Input: part model. Units: mm. Frame: model coordinates. Face numbers are marked on the shaded views. Coordinates: 2 decimals unless noted, no trailing zeros. Loops run counter-clockwise (first coordinate to the right, second up) from the corner with the lowest first, then second, coordinate; pieces in that order, holes last. Notation, with made-up numbers: (25, -26.5) - (34, -26.5) arc R10 ccw to (34, -12.5) - close; hole circle Ø2 at (88, -26). An arc over 180 degrees is marked (long way). Use a Markdown table: item, result. Add a question column.
1. Contact query for flat-ended pins moving along their axis: P1, Ø12.5, axis at x = 163, z = 273, coming from the -Y side; P2, Ø12.5, axis at y = -340.5, z = 255, coming from the -X side; P3, Ø20.5, axis at y = -67.5, z = 149, coming from the +X side; P4, Ø15, axis at x = 212.5, y = -168, coming from the +Z side. Output: stop coordinate, or through.
2. Section query B-B on x = 169.5. Return the cut outline in (y, z).
3. Section query A-A on z = 201.5. Return the cut outline in (x, y), then the cut area to 3 significant figures.
4. Ray query, L1, parallel to Z at x = 201, y = -199; L2, parallel to Y at x = 237.5, z = 107. Return the intervals inside material, ascending. Write a range as [from, to].
5. Draft query along X for the marked faces 1, 2 and 3. Return one class per face: released by +X, released by -X, zero draft, split by the parting line, or undercut.
Autodesk Inventor part; units mm, degrees
ref_plane "YZ Plane" through (0, 0, 0) normal (1, 0, 0) x (0, 1, 0)
ref_plane "XZ Plane" through (0, 0, 0) normal (0, 1, 0) x (-1, 0, 0)
ref_plane "XY Plane" through (0, 0, 0) normal (0, 0, 1) x (1, 0, 0)
sketch "Sketch1" plane through (0, 0, 0) normal (0, 0, 1) x (1, 0, 0)
  line L0 (0, 0) -> (812.8, 0) construction
  line L1 (812.8, 0) -> (812.8, -406.4) construction
  line L2 (812.8, -406.4) -> (0, -406.4) construction
  line L3 (0, -406.4) -> (0, 0) construction
  line L4 (0, 0) -> (406.4, 0)
  line L5 (406.4, 0) -> (406.4, -25.4)
  line L6 (406.4, -25.4) -> (0, -25.4)
  line L7 (0, -25.4) -> (0, 0)
  line L8 (406.4, -25.4) -> (381, -25.4)
  line L9 (381, -25.4) -> (381, -406.4)
  line L10 (381, -406.4) -> (406.4, -406.4)
  line L11 (406.4, -406.4) -> (406.4, -25.4)
  line L12 (381, -406.4) -> (0, -406.4)
  line L13 (0, -406.4) -> (0, -381)
  line L14 (0, -381) -> (381, -381)
  line L15 (381, -381) -> (381, -406.4)
  line L16 (0, -381) -> (25.4, -381)
  line L17 (25.4, -381) -> (25.4, -25.4)
  line L18 (25.4, -25.4) -> (0, -25.4)
  line L19 (0, -25.4) -> (0, -381)
  dimension "d1" = 812.8
  dimension "d5" = 406.4
  dimension "d6" = 25.4
  dimension "d7" = 25.4
  dimension "d8" = 381
  dimension "d9" = 381
  dimension "d10" = 25.4
  dimension "d11" = 25.4
extrude "Extrusion1" add sketch "Sketch1" against normal blind 25.4 contours L6 L9 L14 L17
sketch "Sketch3" plane through (0, 0, 0) normal (0, 0, 1) x (1, 0, 0)
  line L0 (-406.4, 0) -> (406.4, 0) construction
  line L1 (406.4, 0) -> (406.4, -406.4) construction
  line L2 (406.4, -406.4) -> (-406.4, -406.4) construction
  line L3 (-406.4, -406.4) -> (-406.4, 0) construction
  line L4 (406.4, -406.4) -> (406.4, 0)
  line L5 (381, -381) -> (25.4, -381)
  line L6 (25.4, -381) -> (177.8, -381)
  line L7 (177.8, -381) -> (203.2, -381)
  line L8 (177.8, -381) -> (177.8, -355.6)
  line L9 (177.8, -355.6) -> (228.6, -355.6)
  line L10 (228.6, -355.6) -> (228.6, -330.2)
  line L11 (228.6, -330.2) -> (254, -330.2)
  line L12 (254, -330.2) -> (254, -76.2)
  line L13 (254, -76.2) -> (228.6, -76.2)
  line L14 (228.6, -76.2) -> (228.6, -50.8)
  line L15 (228.6, -50.8) -> (177.8, -50.8)
  line L16 (177.8, -50.8) -> (177.8, -76.2)
  line L17 (177.8, -76.2) -> (152.4, -76.2)
  line L18 (152.4, -76.2) -> (152.4, -330.2)
  line L19 (152.4, -330.2) -> (177.8, -330.2)
  line L20 (177.8, -330.2) -> (177.8, -355.6)
  point P0 (0, 0)
  dimension "d36" = 812.8
  dimension "d48" = 152.4
  dimension "d49" = 25.4
  dimension "d50" = 25.4
  dimension "d51" = 50.8
  dimension "d52" = 25.4
  dimension "d53" = 25.4
  dimension "d54" = 254
  dimension "d55" = 25.4
  dimension "d56" = 25.4
  dimension "d57" = 50.8
  dimension "d58" = 25.4
  dimension "d59" = 25.4
  dimension "d60" = 254
  dimension "d61" = 25.4
extrude "Extrusion3" add sketch "Sketch3" along normal blind 393.7
sketch "Sketch4" plane through (381, -381, 0) normal (1, 0, 0) x (0, 0, -1)
  line L0 (0, 355.6) -> (25.4, 355.6)
  line L1 (153.8842, -0.5875) -> (0, -0.5875)
  line L2 (0, -0.5875) -> (0, 355.6)
  line L3 (0, 355.6) -> (153.8842, 355.6)
  line L4 (153.8842, 355.6) -> (153.8842, -0.5875)
  point P0 (0, 381)
extrude "Extrusion4" cut sketch "Sketch4" against normal blind 393.7
sketch "Sketch5" plane through (0, 0, 393.7) normal (0, 0, 1) x (1, 0, 0)
  line L0 (177.8, -50.8) -> (177.8, -76.2)
  line L1 (228.6, -355.6) -> (228.6, -330.2)
  line L2 (177.8, -76.2) -> (228.6, -76.2)
  line L3 (228.6, -76.2) -> (228.6, -330.2)
  line L4 (228.6, -330.2) -> (177.8, -330.2)
  line L5 (177.8, -330.2) -> (177.8, -76.2)
  point P0 (0, 0)
extrude "Extrusion5" cut sketch "Sketch5" against normal blind 2.54
properties part number "JukeBox CD Player"
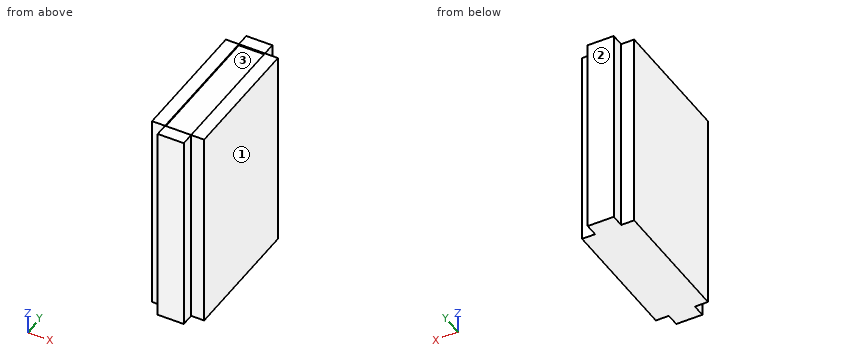
Resolved:
| question | item | result |
|---|---|---|
| 1 | P1 | y = -330.2 |
| 1 | P2 | x = 177.8 |
| 1 | P3 | x = 254 |
| 1 | P4 | z = 391.16 |
| 2 | outline | (-330.2, 0) - (-76.2, 0) - (-76.2, 393.7) - (-330.2, 393.7) - close |
| 3 | outline | (152.4, -330.2) - (177.8, -330.2) - (177.8, -355.6) - (228.6, -355.6) - (228.6, -330.2) - (254, -330.2) - (254, -76.2) - (228.6, -76.2) - (228.6, -50.8) - (177.8, -50.8) - (177.8, -76.2) - (152.4, -76.2) - close |
| 3 | area | 28,400 mm² |
| 4 | L1 | [0, 391.16] |
| 4 | L2 | [-330.2, -76.2] |
| 5 | face 1 | released by +X |
| 5 | face 2 | zero draft |
| 5 | face 3 | undercut |
